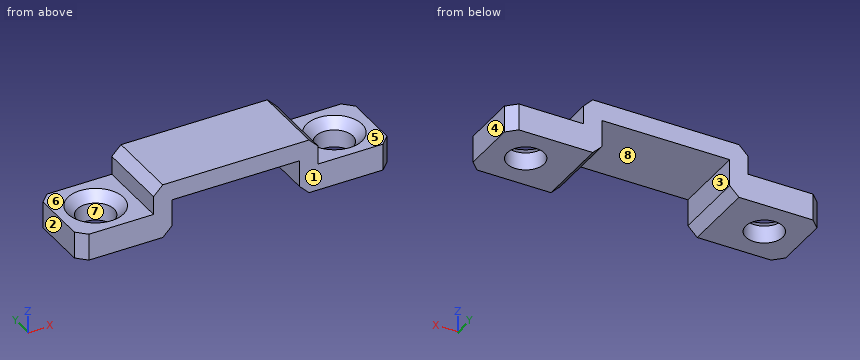
from build123d import *

# Parameters (mm, degrees)
F0_W     = 2
F0_H     = 8
F0_W_2   = 13.8
F1_DEPTH = 2
F0_R     = 2
F2_DEPTH = 3.9
F3_DEPTH = 1
F4_SIZE  = 1


with BuildPart() as f1:
    # F0 (on Top) → F1 (new body)
    with BuildSketch(Plane.XY):
        with Locations((-7.9, 0)):
            Rectangle(F0_W, F0_H)
        Rectangle(F0_W_2, F0_H)
        with Locations((7.9, 0)):
            Rectangle(F0_W, F0_H)
    extrude(amount=F1_DEPTH)

    # F0 (on Top) → F2 (join)
    with BuildSketch(Plane.XY):
        with Locations((-7.9, 0)):
            Rectangle(F0_W, F0_H)
        Polygon((-16.9, -4), (-8.9, -4), (-8.9, 4), (-16.9, 4), (-16.9, 0), align=None)
        with Locations((-12.9, 0)):
            Circle(F0_R, mode=Mode.SUBTRACT)
        with Locations((7.9, 0)):
            Rectangle(F0_W, F0_H)
        Polygon((8.9, 4), (8.9, -4), (16.9, -4), (16.9, 0), (16.9, 4), align=None)
        with Locations((12.9, 0)):
            Circle(F0_R, mode=Mode.SUBTRACT)
    extrude(amount=-F2_DEPTH)

    # F0 (on Top) → F3 (cut)
    with BuildSketch(Plane.XY):
        Polygon((-16.9, -4), (-8.9, -4), (-8.9, 4), (-16.9, 4), (-16.9, 0), align=None)
        with Locations((-12.9, 0)):
            Circle(F0_R, mode=Mode.SUBTRACT)
        Polygon((8.9, 4), (8.9, -4), (16.9, -4), (16.9, 0), (16.9, 4), align=None)
        with Locations((12.9, 0)):
            Circle(F0_R, mode=Mode.SUBTRACT)
    extrude(amount=-F3_DEPTH, mode=Mode.SUBTRACT)

    # F4
    f4_edges = [f1.edges().sort_by_distance(p)[0] for p in [
        (-8.9, 0, 2),
        (8.9, 0, 2),
        (-6.9, 0, -3.9),
        (-14.9, 0, -1),
        (10.9, 0, -1),
        (6.9, 0, -3.9),
        (-16.9, -4, -2.45),
        (-16.9, 4, -2.45),
        (16.9, -4, -2.45),
        (16.9, 4, -2.45),
    ]]
    chamfer(f4_edges, length=F4_SIZE)


solid = f1.part
The model under review builds one solid part; all positions refer to its coordinate system, in mm. Face numbers are marked on the shaded views. A direction names the side the tool comes from. Round coordinates to 2 decimals unless told otherwise and drop trailing zeros. Loops run counter-clockwise (first coordinate to the right, second up) from the corner with the lowest first, then second, coordinate; pieces in that order, holes last. Notation, with made-up numbers: (41.5, -38.75) -> (46.5, -38.75) arc R24 ccw to (46.5, -6.75) -> close; hole circle Ø11 at (-37, 17.5). An arc over 180 degrees is marked (long way). Answer as CSV lines item,"result".
1) Tool access review of the marked faces 5, 6, 7 and 8: name each direction out of +Z, -Z, +X, -X, +Y, -Y from which nothing blocks a thin tool from reaching the whole face with its end or side.
Geometry results:
face 5,"+Z, +X, +Y, -Y"
face 6,"+Z, -X, +Y, -Y"
face 7,"+Z, -Z"
face 8,"-Z, +Y, -Y"
2) To check wall thickness, follow line 1 along Y through (x, z) = (-12.9, -3.15); line 2 along X through (y, z) = (0.75, -0.4); line 3 along X through (y, z) = (-1.5, -1.25). State the ranges of each line that lie inside material, in increasing order. Write a range as from..to.
Geometry results:
line 1,"y = -4..-2, 2..4"
line 2,"x = -8.9..-6.9, 6.9..8.9"
line 3,"x = -16.9..-15.2, -10.6..-6.9, 6.9..10.6, 15.2..16.9"
3) For P1, Ø1, axis at y = -1.5, z = 0.5, coming from the -X side; P2, Ø1.5, axis at x = -12.5, y = 2, coming from the +Z side; P3, Ø4, axis at x = 14, y = 1, coming from the +Z side, all flat-tipped, find the tip position at first contact; note any pin that passes through.
Geometry results:
P1,"stops at x = -8.9"
P2,"stops at z = -1.21"
P3,"stops at z = -1"
4) Add section A-A on z = -2.6. Write out the cut boundary in (x, y).
Geometry results:
outline,"(-16.9, -3) -> (-15.9, -4) -> (-6.9, -4) -> (-6.9, 4) -> (-15.9, 4) -> (-16.9, 3) -> close; (6.9, -4) -> (15.9, -4) -> (16.9, -3) -> (16.9, 3) -> (15.9, 4) -> (6.9, 4) -> close; hole circle Ø4 at (-12.9, 0); hole circle Ø4 at (12.9, 0)"
5) Draft analysis for pull direction X (two halves, no side actions). For the marked faces 1, 2, 3 and 4, state which applies: pulls with the +X half, pulls with the -X half, needs draft (parallel to the pull), parting line crosses it, or undercut.
Geometry results:
face 1,"needs draft"
face 2,"pulls with the -X half"
face 3,"undercut"
face 4,"pulls with the +X half"
6) Add section D-D on z = -1.3. Write out the cut boundary in (x, y), plus the area to 3 significant figures.
Geometry results:
outline,"(-16.9, -3) -> (-15.9, -4) -> (-6.9, -4) -> (-6.9, 4) -> (-15.9, 4) -> (-16.9, 3) -> close; (6.9, -4) -> (15.9, -4) -> (16.9, -3) -> (16.9, 3) -> (15.9, 4) -> (6.9, 4) -> close; hole circle Ø5.4 at (-12.9, 0); hole circle Ø5.4 at (12.9, 0)"
area,"112 mm²"
7) Add section B-B on x = 12.9. Write out the cut boundary in (y, z), plus the area to 3 significant figures.
Geometry results:
outline,"(-4, -3.9) -> (-2, -3.9) -> (-2, -2) -> (-3, -1) -> (-4, -1) -> close; (2, -3.9) -> (4, -3.9) -> (4, -1) -> (3, -1) -> (2, -2) -> close"
area,"10.6 mm²"
8) Add section C-C on y = 0. Write out the cut boundary in (x, z).
Geometry results:
outline,"(-16.9, -3.9) -> (-14.9, -3.9) -> (-14.9, -2) -> (-15.9, -1) -> (-16.9, -1) -> close; (-10.9, -3.9) -> (-7.9, -3.9) -> (-6.9, -2.9) -> (-6.9, 0) -> (6.9, 0) -> (6.9, -2.9) -> (7.9, -3.9) -> (10.9, -3.9) -> (10.9, -2) -> (9.9, -1) -> (8.9, -1) -> (8.9, 1) -> (7.9, 2) -> (-7.9, 2) -> (-8.9, 1) -> (-8.9, -1) -> (-9.9, -1) -> (-10.9, -2) -> close; (14.9, -3.9) -> (16.9, -3.9) -> (16.9, -1) -> (15.9, -1) -> (14.9, -2) -> close"
